Autodesk Inventor part; units mm, degrees
ref_plane "YZ Plane" through (0, 0, 0) normal (1, 0, 0) x (0, 1, 0)
ref_plane "XZ Plane" through (0, 0, 0) normal (0, 1, 0) x (-1, 0, 0)
ref_plane "XY Plane" through (0, 0, 0) normal (0, 0, 1) x (1, 0, 0)
sketch "Sketch1" plane through (0, 0, 0) normal (0, 0, 1) x (1, 0, 0)
  circle A0 centre (0, 0) radius 1.5875
  circle A1 centre (0, 0) radius 4.7625
  dimension "d1" = 3.175
  dimension "d2" = 9.525
extrude "Extrusion1" add sketch "Sketch1" along normal mid plane 12.7
sketch "Sketch2" plane through (0, 0, 0) normal (0, 1, 0) x (-1, 0, 0)
  circle A0 centre (0, 3.175) radius 1.5875
  circle A1 centre (0, -3.175) radius 1.6216
  point P0 (0, 0)
  dimension "d5" = 3.175
  dimension "d6" = 3.175
  dimension "d7" = 3.175
extrude "Extrusion2" cut sketch "Sketch2" along normal blind 7.9375
properties part number "coupler" material "ABS Plastic"
The listing builds one solid part. Answer for the finished solid, in the listing's coordinates (mm). A direction names the side the tool comes from. Coordinates: 2 decimals unless noted, no trailing zeros. Loops run counter-clockwise (first coordinate to the right, second up) from the corner with the lowest first, then second, coordinate; pieces in that order, holes last. Notation, with made-up numbers: M -26.5,79 L -1.5,79 A30 ccw -1.5,112 Z; hole C -22.5,47.5 d3. An arc over 180 degrees is marked long. Answer as CSV lines item,"result". Start each with the question number.
(1) The part is cut by section C-C (z = 0.5). Give the vertices of the cut face in (x, y) (1 decimal).
(2) The mould has two halves that part along X. Classify faces 3 (the cylindrical face through (1.62, 2.88, -3.25)), 4 (the cylindrical face through (-0.62, -4.72, -0.09)), 5 (the flat face through (2, 0, 6.35)): pulls with the +X half, pulls with the -X half, needs draft (parallel to the pull), parting line crosses it, or undercut.
(3) For faces 1 (the cylindrical face through (1.586, 2.878, 3.105)), 2 (the flat face through (2, 0, -6.35)), determine the directions among +Z, -Z, +X, -X, +Y, -Y from which every point of the face is accessible in a straight line to the end or side of a thin tool.
(4) Given pin 1 (4 mm diameter, centred on x = -2.5, z = 2, fed in from +Y); pin 2 (2.5 mm diameter, centred on x = 0, z = 3.175, fed in from +Y), each flat-ended and moving along its own axis, determine where each tip first touches the part or whether it passes through.
(5) Find the intervals of material crossed by L1, parallel to Z at x = 0, y = 3.45; L2, parallel to Y at x = 0, z = -1.5; L3, parallel to Z at x = 1, y = 3, in increasing order. Write a range as [from, to].
(6) The part is cut by section B-B (y = -0.5). Give the vertices of the cut face in (x, z).
(7) The part is cut by section A-A (x = 0). Give the vertices of the cut face in (y, z), and give its area (3 significant figures).
Determined:
1,outline,"C 0,0 d9.5; hole C 0,0 d3.2"
2,face 3,"undercut"
2,face 4,"parting line crosses it"
2,face 5,"needs draft"
3,face 1,"+Y"
3,face 2,"-Z, +X, -X, +Y, -Y"
4,pin 1,"y = 4.73"
4,pin 2,"y = -0.98"
5,L1,"[-6.35, -4.8], [-1.55, 1.59], [4.76, 6.35]"
5,L2,"[-4.76, -1.59], [1.59, 4.76]"
5,L3,"[-6.35, -4.45], [-1.9, 1.94], [4.41, 6.35]"
6,outline,"M -4.74,-6.35 L -1.51,-6.35 L -1.51,6.35 L -4.74,6.35 Z; M 1.51,-6.35 L 4.74,-6.35 L 4.74,6.35 L 1.51,6.35 Z"
7,outline,"M -4.76,-6.35 L -1.59,-6.35 L -1.59,6.35 L -4.76,6.35 Z; M 1.59,-6.35 L 4.76,-6.35 L 4.76,-4.8 L 1.59,-4.8 Z; M 1.59,-1.55 L 4.76,-1.55 L 4.76,1.59 L 1.59,1.59 Z; M 1.59,4.76 L 4.76,4.76 L 4.76,6.35 L 1.59,6.35 Z"
7,area,"60.3 mm2"
